For this review, use the dimensioned drawing (mm, ordinates from the lowest corner) and the shaded views. A direction names the side the tool comes from. Give positions to 0.01 mm unless a question says otherwise; leave off trailing zeros. Loops run counter-clockwise (first coordinate to the right, second up) from the corner with the lowest first, then second, coordinate; pieces in that order, holes last. Notation, with made-up numbers: M 15.25,53 L 62.25,53 A9 cw 62.25,65 Z; hole C -36.75,64.5 d3. An arc over 180 degrees is marked long. Use CSV: the item, a comma, the result in double quotes. Start each with the question number.
1. Take a section at B-B, the plane x = 53. Write out the cut boundary in (y, z).
2. Take a section at A-A, the plane z = 11.5. Write out the cut boundary in (x, y).
3. Take a section at D-D, the plane x = 36.5. Write out the cut boundary in (y, z), and give its area (3 significant figures).
4. Insertion check: P1, Ø22, axis at x = 12, z = 12.5, coming from the +Y side; P2, Ø1.5, axis at x = 29.5, z = 25, coming from the +Y side; P3, Ø8, axis at x = 67, z = 38, coming from the +Y side. Each pin has a flat end and moves straight along its axis. Give the tip position at first contact, or say it passes through.
5. To check wall thickness, follow line 1 (Y direction, x = 6, z = 30); line 2 (Y direction, x = 41, z = 40); line 3 (Z direction, x = 21, y = 24.5). State the ranges of each line that lie inside material, in increasing order. Write a range as [from, to].
6. Tool access review of the marked faces 1, 2, 3 and 4: name each direction out of +Z, -Z, +X, -X, +Y, -Y from which nothing blocks a thin tool from reaching the whole face with its end or side.
7. Take a section at C-C, the plane y = 42. Write out the cut boundary in (x, z).
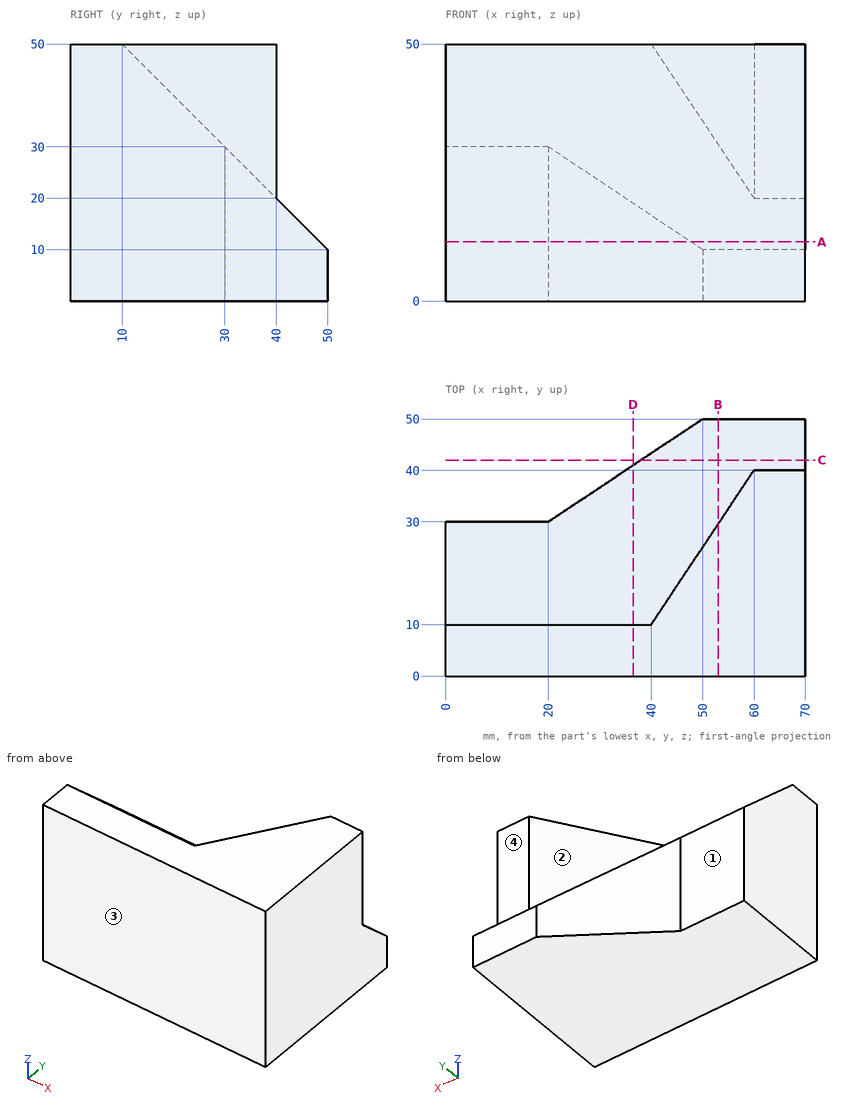
Result set:
1,outline,"M 0,0 L 50,0 L 50,10 L 29.5,30.5 L 29.5,50 L 0,50 Z"
2,outline,"M 0,0 L 70,0 L 70,48.5 L 47.75,48.5 L 20,30 L 0,30 Z"
3,outline,"M 0,0 L 41,0 L 41,19 L 10,50 L 0,50 Z"
3,area,"1,570 mm2"
4,P1,"y = 32"
4,P2,"y = 35.75"
4,P3,"y = 40"
5,line 1,"[0, 30]"
5,line 2,"[0, 20]"
5,line 3,"[0, 35.5]"
6,face 1,"+Z, -Z, -X, +Y"
6,face 2,"+Z, -X, +Y"
6,face 3,"+Z, -Z, +X, -X, -Y"
6,face 4,"+Z, +X, -X, +Y"
7,outline,"M 38,0 L 70,0 L 70,18 L 38,18 Z"
